Answer from the drawing. Dimensions are ordinates in mm from the lowest x, y and z of the part. A direction names the side the tool comes from. Round coordinates to 2 decimals unless told otherwise and drop trailing zeros. Loops run counter-clockwise (first coordinate to the right, second up) from the corner with the lowest first, then second, coordinate; pieces in that order, holes last.
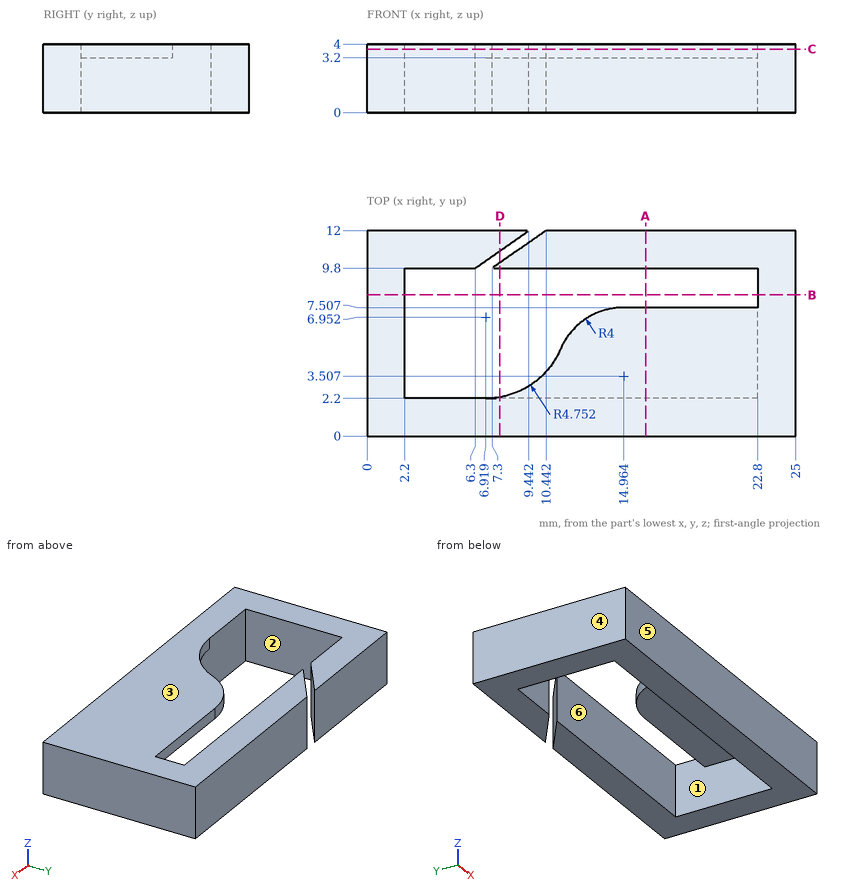
1. Determine the mould class of the marked faces 4, 5 and 6 for opening direction Y: +Y half, -Y half, draft (parallel to the pull), parting line (faces both ways), or undercut.
Answer key:
face 4: draft
face 5: -Y half
face 6: undercut
2. Find section D-D (x = 7.75). Give the number of separate pieces and of enclosed holes in the cut face.
Answer key:
separate pieces: 3
enclosed holes: 0
3. Consider probe 1 along Y at (x, z) = (22.5, 0.3); probe 2 along X at (y, z) = (9, 0.6); probe 3 along Y at (x, z) = (18, 3.4). Determine where each line is inside the solid, lowest interval first.
Answer key:
probe 1: y = 0 to 2.2, 9.8 to 12
probe 2: x = 0 to 2.2, 22.8 to 25
probe 3: y = 0 to 7.51, 9.8 to 12
4. Given pin 1 (2.5 mm diameter, centred on x = 17.5, y = 4, fed in from -Z); pin 2 (1.5 mm diameter, centred on y = 8.5, z = 2, fed in from -X), each flat-ended and moving along its own axis, determine where each tip first touches the part or whether it passes through.
Answer key:
pin 1: stops at z = 3.2
pin 2: stops at x = 0
5. Find section A-A (x = 16.25). Write down the section's boundary in (y, z).
Answer key:
outline: (0, 0) - (2.2, 0) - (2.2, 3.2) - (7.51, 3.2) - (7.51, 4) - (0, 4) - close; (9.8, 0) - (12, 0) - (12, 4) - (9.8, 4) - close
6. Find section C-C (z = 3.7). Write down the section's boundary in (x, y) (1 decimal).
Answer key:
outline: (0, 0) - (25, 0) - (25, 12) - (10.4, 12) - (7.3, 9.8) - (22.8, 9.8) - (22.8, 7.5) - (15, 7.5) arc R4 ccw to (11.3, 5.1) arc R4.8 cw to (6.9, 2.2) - (2.2, 2.2) - (2.2, 9.8) - (6.3, 9.8) - (9.4, 12) - (0, 12) - close
7. Which of the six approach directions +Z, -Z, +X, -X, +Y, -Y give full straight-line access (tool end or side, diameter ignored) to the marked faces 1, 2 and 3?
Answer key:
face 1: -Z
face 2: +Z, -Z
face 3: +Z, +X, -X, +Y, -Y
8. Find section B-B (y = 8.25). Write down the section's boundary in (x, z).
Answer key:
outline: (0, 0) - (2.2, 0) - (2.2, 4) - (0, 4) - close; (22.8, 0) - (25, 0) - (25, 4) - (22.8, 4) - close
